Verification items for the finished model (mm, model axes). Face numbers are marked on the shaded views. A direction names the side the tool comes from. Round coordinates to 2 decimals unless told otherwise and drop trailing zeros. Order: outer loops, then holes, each group sorted by start corner. A loop starts at its lowest first (then second) coordinate and runs counter-clockwise, first axis right, second up. Notation, with made-up numbers: (77.5, 3.5) -> (87.5, 3.5) arc R14 ccw to (87.5, 22.5) -> close; hole circle Ø9 at (17, 80.25). An arc over 180 degrees is marked (long way). Put each result on its own line as item: value.
```python
from build123d import *

# Parameters (mm, degrees)
F1_DEPTH     = 140.081
F2_DEPTH     = 140.0048
F3_DEPTH     = 68.5038
F4_DEPTH     = 68.5038
F5_T         = -5.08
F6_T         = 2.54
F6_T3_DEPTH  = 142.0876
F6_T5_DEPTH  = 71.08
F6_T7_DEPTH  = 275.0058
F6_T9_DEPTH  = 47.0194652776
F6_T11_DEPTH = 76.581
F6_T13_DEPTH = 9.2884577092
F6_T15_DEPTH = 76.6572
F6_T17_DEPTH = 125.7681103512
F6_T19_DEPTH = 47.0149573841
F6_T21_DEPTH = 66.8341103512
F6_T23_DEPTH = 47.0149573841
F6_T25_DEPTH = 9.2884593969
F6_T27_DEPTH = 42.1653521873
F6_T29_DEPTH = 42.16567527


# Not quite as in the source:
# - a shell that OpenCascade refuses in one call is made with other operations: the cavity is built on its own and cut out


with BuildPart() as f1:
    # F0 (on Front) → F1 (new body)
    with BuildSketch(Plane.XZ):
        Polygon((-72.5043, 57.5), (-33, 17.5), (0, 17.5), (33, 17.5), (72.4957, 57.5), align=None)
    extrude(amount=F1_DEPTH)

    # F0 (on Front) → F2 (join)
    with BuildSketch(Plane.XZ):
        Polygon((-72.5043, 57.5), (-33, 17.5), (0, 17.5), (33, 17.5), (72.4957, 57.5), align=None)
    extrude(amount=-F2_DEPTH)

    # F0 (on Front) → F3 (join)
    with BuildSketch(Plane.XZ):
        Polygon((-33, 17.5), (-33, -17.5), (33, -17.5), (33, 17.5), (0, 17.5), align=None)
    extrude(amount=-F3_DEPTH)

    # F0 (on Front) → F4 (join)
    with BuildSketch(Plane.XZ):
        Polygon((-33, 17.5), (-33, -17.5), (33, -17.5), (33, 17.5), (0, 17.5), align=None)
    extrude(amount=F4_DEPTH)

    # F5
    f5_openings = [f1.faces().sort_by_distance(p)[0] for p in [
        (0, 0, -17.5),
    ]]
    offset(amount=F5_T, openings=f5_openings, kind=Kind.INTERSECTION)

    # F6: shell of thickness 2.54, made by hand


with BuildPart() as f6_core1:
    # F6_t2: copy of F1
    add(f1.part)

    # the walls: a layer under each face that stays
    f6_faces = [f6_core1.faces().sort_by_distance(p)[0] for p in [
        (-52.75215, -0.0381, 37.5),
        (-0.0043, 140.0048, 37.5),
        (52.74785, -0.0381, 37.5),
        (33, 0, 0),
        (0, -68.5038, 0),
        (0, 68.5038, 0),
        (0, 104.2543, 17.5),
        (-33, 0, 0),
        (0, -104.2924, 17.5),
        (-0.0043, -140.081, 37.5),
        (-28.2857142857, 58.7175428571, -17.5),
        (-44.1337126804, -0.0381, 36.002837635),
        (-0.0033701852, 134.9248, 37.5),
        (44.1303424952, -0.0381, 36.0026760937),
        (27.92, 0, 1.0426760937),
        (28.4128154651, -63.4238, 21.0826760937),
        (0, -63.4238, 2.54),
        (-29.3986087804, -63.4238, 22.0809458783),
        (28.4128154651, 63.4238, 21.0826760937),
        (0, 63.4238, 2.54),
        (-29.3986087804, 63.4238, 22.0809458783),
        (-0.0001623852, 99.1743, 22.58),
        (-27.92, 0, 1.042837635),
        (-0.0001623852, -99.2124, 22.58),
        (-0.0033701852, -135.001, 37.5),
        (-0.0033701852, -0.0381, 52.42),
    ]]
    thicken(f6_faces, amount=-F6_T, mode=Mode.SUBTRACT)

    # F6_s4 → F6_t3 (cut)
    with BuildSketch(Plane.XZ.offset(-71.0438)):
        Polygon((-33.0434721427, 17.4821518164), (-31.192785733, 19.2848183642), (-30.46, 18.542837635), (-30.46, 17.5), align=None)
        Polygon((33.0434740854, 17.4821537837), (31.1925914624, 19.2846216345), (30.46, 18.5426760937), (30.46, 17.5), align=None)
    extrude(amount=F6_T3_DEPTH, mode=Mode.SUBTRACT)

    # F6_s6 → F6_t5 (cut)
    with BuildSketch(Plane.YZ.offset(-35.54)):
        Polygon((-68.5292, 17.4746), (-65.9638, 17.5), (-65.9638, 20.04), (-68.5038, 20.04), align=None)
        Polygon((68.5292, 17.4746), (65.9638, 17.5), (65.9638, 20.04), (68.5038, 20.04), align=None)
    extrude(amount=F6_T5_DEPTH, mode=Mode.SUBTRACT)

    # F6_s8 → F6_t7 (cut)
    with BuildSketch(Plane.XZ.offset(-137.4648)):
        Polygon((-60.3293532181, 52.4124481836), (-62.1546396278, 50.6351816358), (-66.4258626804, 54.96), (-60.3474253608, 54.96), align=None)
        Polygon((60.322610905, 52.4124462163), (62.148093528, 50.6353783655), (66.4181924952, 54.96), (60.3406849904, 54.96), align=None)
    extrude(amount=F6_T7_DEPTH, mode=Mode.SUBTRACT)

    # F6_s10 → F6_t9 (cut)
    with BuildSketch(Plane(origin=(-57.7902488571, 0, 58.5154009635), x_dir=(0, 1, 0), z_dir=(0.7026843954, 0, -0.7115016799))):
        Polygon((134.8994, -6.0771785187), (134.9248, -8.6425785187), (137.4648, -8.6425785187), (137.4648, -6.1025785187), align=None)
        Polygon((-134.9756, -6.0771785187), (-135.001, -8.6425785187), (-137.541, -8.6425785187), (-137.541, -6.1025785187), align=None)
    extrude(amount=F6_T9_DEPTH, mode=Mode.SUBTRACT)

    # F6_s12 → F6_t11 (cut)
    with BuildSketch(Plane.XZ.offset(-137.4648)):
        Polygon((-30.8591454181, 22.6232481836), (-32.6844318278, 20.7951816358), (-31.9386087804, 20.04), (-30.8772175608, 20.04), align=None)
        Polygon((30.858818705, 22.6232462163), (32.684301328, 20.7953783655), (31.9384463952, 20.04), (30.8768927904, 20.04), align=None)
    extrude(amount=F6_T11_DEPTH, mode=Mode.SUBTRACT)

    # F6_s14 → F6_t13 (cut)
    with BuildSketch(Plane(origin=(-28.3200410571, 0, 28.6754009635), x_dir=(0, 1, 0), z_dir=(0.7026843954, 0, -0.7115016799))):
        Polygon((63.3984, -6.0771785187), (63.4238, -8.6425785187), (65.9638, -8.6425785187), (65.9638, -6.1025785187), align=None)
        Polygon((-63.3984, -6.0771785187), (-63.4238, -8.6425785187), (-65.9638, -8.6425785187), (-65.9638, -6.1025785187), align=None)
    extrude(amount=F6_T13_DEPTH, mode=Mode.SUBTRACT)

    # F6_s16 → F6_t15 (cut)
    with BuildSketch(Plane.XZ.offset(60.8838)):
        Polygon((-30.8591454181, 22.6232481836), (-32.6844318278, 20.7951816358), (-31.9386087804, 20.04), (-30.8772175608, 20.04), align=None)
        Polygon((30.858818705, 22.6232462163), (32.684301328, 20.7953783655), (31.9384463952, 20.04), (30.8768927904, 20.04), align=None)
    extrude(amount=F6_T15_DEPTH, mode=Mode.SUBTRACT)

    # F6_s18 → F6_t17 (cut)
    with BuildSketch(Plane.YZ.offset(-62.8874253608)):
        Polygon((134.8994, 52.3946), (137.4648, 52.42), (137.4648, 54.96), (134.9248, 54.96), align=None)
        Polygon((-134.9756, 52.3946), (-137.541, 52.42), (-137.541, 54.96), (-135.001, 54.96), align=None)
    extrude(amount=F6_T17_DEPTH, mode=Mode.SUBTRACT)

    # F6_s20 → F6_t19 (cut)
    with BuildSketch(Plane(origin=(57.7800845012, 0, 58.5178482733), x_dir=(0, 1, 0), z_dir=(-0.7026069427, 0, -0.7115781644))):
        Polygon((134.8994, 6.0810579283), (137.4648, 6.1064579283), (137.4648, 8.6464579283), (134.9248, 8.6464579283), align=None)
    extrude(amount=F6_T19_DEPTH, mode=Mode.SUBTRACT)

    # F6_s22 → F6_t21 (cut)
    with BuildSketch(Plane.YZ.offset(-33.4172175608)):
        Polygon((134.8994, 22.6054), (137.4648, 22.58), (137.4648, 20.04), (134.9248, 20.04), align=None)
        Polygon((-134.9756, 22.6054), (-135.001, 20.04), (-137.541, 20.04), (-137.541, 22.58), align=None)
    extrude(amount=F6_T21_DEPTH, mode=Mode.SUBTRACT)

    # F6_s24 → F6_t23 (cut)
    with BuildSketch(Plane(origin=(24.7470490323, 0, 25.0630311981), x_dir=(0, 1, 0), z_dir=(0.7026069427, 0, 0.7115781644))):
        Polygon((-134.9756, -6.0810579283), (-135.001, -8.6464579283), (-137.541, -8.6464579283), (-137.541, -6.1064579283), align=None)
    extrude(amount=F6_T23_DEPTH, mode=Mode.SUBTRACT)

    # F6_s26 → F6_t25 (cut)
    with BuildSketch(Plane(origin=(21.7901562419, 0, 22.0683833854), x_dir=(0, 1, 0), z_dir=(0.7026069427, 0, 0.7115781644))):
        Polygon((-63.3984, -6.0810579283), (-63.4238, -8.6464579283), (-65.9638, -8.6464579283), (-65.9638, -6.1064579283), align=None)
        Polygon((63.3984, -6.0810579283), (63.4238, -8.6464579283), (65.9638, -8.6464579283), (65.9638, -6.1064579283), align=None)
    extrude(amount=F6_T25_DEPTH, mode=Mode.SUBTRACT)

    # F6_s28 → F6_t27 (cut)
    with BuildSketch(Plane.XY.offset(-20.04)):
        Polygon((27.8946, 63.3984), (30.46, 63.4238), (30.46, 65.9638), (27.92, 65.9638), align=None)
        Polygon((27.8946, -63.3984), (30.46, -63.4238), (30.46, -65.9638), (27.92, -65.9638), align=None)
    extrude(amount=F6_T27_DEPTH, mode=Mode.SUBTRACT)

    # F6_s30 → F6_t29 (cut)
    with BuildSketch(Plane.XY.offset(-20.04)):
        Polygon((-27.8946, -63.3984), (-27.92, -65.9638), (-30.46, -65.9638), (-30.46, -63.4238), align=None)
        Polygon((-27.8946, 63.3984), (-27.92, 65.9638), (-30.46, 65.9638), (-30.46, 63.4238), align=None)
    extrude(amount=F6_T29_DEPTH, mode=Mode.SUBTRACT)


with BuildPart() as f1_1:
    add(f1.part)

    # what is left inside the walls is the cavity
    f6_cavity = [f6_core1.part.solids().sort_by_distance(p)[0] for p in [
        (-0.004108, -45.8724, 57.4746),
    ]]
    add(f6_cavity, mode=Mode.SUBTRACT)


solid = f1_1.part
```
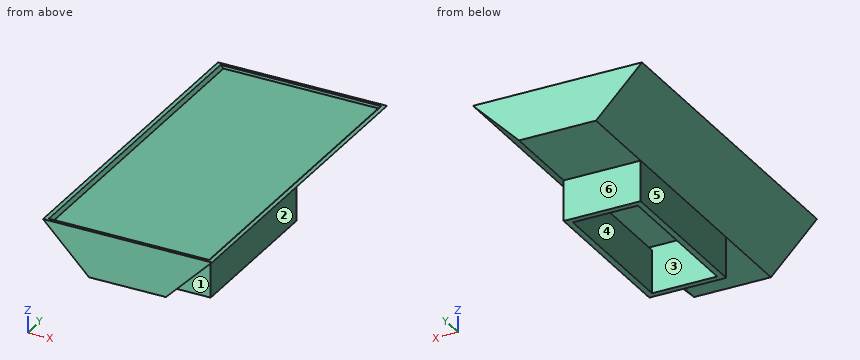
Item 1: Sectioned sample at C-C, the plane y = -18. Record the boundary of the cut face in (x, z).
Geometry check:
outline: (-72.5, 57.5) -> (-33, 17.5) -> (-33, -17.5) -> (-27.92, -17.5) -> (-27.92, 19.59) -> (-60.35, 52.42) -> (60.34, 52.42) -> (27.92, 19.59) -> (27.92, -17.5) -> (33, -17.5) -> (33, 17.5) -> (72.5, 57.5) -> (68.93, 57.5) -> (66.42, 54.96) -> (-66.43, 54.96) -> (-68.93, 57.5) -> close
Item 2: Sectioned sample at D-D, the plane x = 11.5. Record the boundary of the cut face in (y, z), then the cut area to 3 significant figures.
Geometry check:
outline: (-140.08, 17.5) -> (-68.5, 17.5) -> (-68.5, -17.5) -> (-63.42, -17.5) -> (-63.42, 22.58) -> (-135, 22.58) -> (-135, 52.42) -> (134.92, 52.42) -> (134.92, 22.58) -> (63.42, 22.58) -> (63.42, -17.5) -> (68.5, -17.5) -> (68.5, 17.5) -> (140, 17.5) -> (140, 57.5) -> (137.46, 57.5) -> (137.46, 54.96) -> (-137.54, 54.96) -> (-137.54, 57.5) -> (-140.08, 57.5) -> close
area: 2,160 mm2
Item 3: Release check for a two-part mould opening along X. For the marked faces 1, 2 and 3 record: pulls with the +X half, pulls with the -X half, needs draft (parallel to the pull), parting line crosses it, or undercut.
Geometry check:
face 1: needs draft
face 2: pulls with the +X half
face 3: undercut
Item 4: Material ranges on line 1 along Y through (x, z) = (-39, 47); line 2 along Y through (x, z) = (19.5, -4); line 3 along Z through (x, y) = (29.5, -109.5), recorded low to high.
Geometry check:
line 1: -140.08 to -135, 134.92 to 140
line 2: -68.5 to -63.42, 63.42 to 68.5
line 3: 17.5 to 22.58, 52.42 to 54.96
Item 5: Tool access check on the marked faces 4, 5 and 6. Record the directions out of +Z, -Z, +X, -X, +Y, -Y that give a thin tool (end or side, any length) a straight path to the whole face; none if there is none.
Geometry check:
face 4: -Z
face 5: -Z, -X, +Y, -Y
face 6: -Z, +X, -X, +Y
Item 6: Sectioned sample at A-A, the plane y = 102. Record the boundary of the cut face in (x, z).
Geometry check:
outline: (-72.5, 57.5) -> (-33, 17.5) -> (33, 17.5) -> (72.5, 57.5) -> (68.93, 57.5) -> (66.42, 54.96) -> (-66.43, 54.96) -> (-68.93, 57.5) -> close; hole (-60.35, 52.42) -> (-30.88, 22.58) -> (30.88, 22.58) -> (60.34, 52.42) -> close
Item 7: Depth check by flat-ended pin: pin 1 Ø20 at (x, y) = (-2.5, 111.5) entering from -Z; pin 2 Ø11 at (y, z) = (-12, 4) entering from +X; pin 3 Ø12 at (x, z) = (3, -4) entering from -Y; pin 4 Ø2 at (x, z) = (40.5, 22) entering from +Y. Enter the tip coordinate at first touch or a pass-through.
Geometry check:
pin 1: z = 17.5
pin 2: x = 33
pin 3: y = -68.5
pin 4: through
Item 8: Sectioned sample at B-B, the plane z = -12. Record the boundary of the cut face in (x, y).
Geometry check:
outline: (-33, -68.5) -> (33, -68.5) -> (33, 68.5) -> (-33, 68.5) -> close; hole (-27.92, -63.42) -> (27.92, -63.42) -> (27.92, 63.42) -> (-27.92, 63.42) -> close
